Design review of the part built by this model. Coordinates are the model's own, in mm. Face numbers are marked on the shaded views. A direction names the side the tool comes from. Coordinates: 2 decimals unless noted, no trailing zeros. Write each loop counter-clockwise with the first axis right and the second up, starting at its lowest first coordinate (ties: lowest second). Pieces come first, ordered by that corner, then holes.
Q1. For probe 1 along Y at (x, z) = (0, -0.25); probe 2 along Y at (x, z) = (0, 6); probe 3 along Z at (x, y) = (1.5, 6), list the stretches that pass through material, from the lowest coordinate up.
Q2. Take a section at D-D (x = 3.5). Give the boundary of the cut face in (y, z).
Q3. Take a section at C-C (z = 6.25). Give the boundary of the cut face in (x, y).
Q4. Take a section at A-A (x = 0). Give the boundary of the cut face in (y, z), and give its area (3 significant figures).
Q5. Mouldability with a two-part tool opening along Y and no side actions: class the marked faces 3, 4 and 5 as pulls with the +Y half, pulls with the -Y half, needs draft (parallel to the pull), parting line crosses it, or undercut.
Q6. Machinability: for the marked faces 1 and 2, which of the approach directions +Z, -Z, +X, -X, +Y, -Y give a long, thin tool a straight path to every point of the face, cutting with its end or side? Answer none if there is none.
Q7. Insertion check: pin 1 (1.5 mm diameter, centred on x = 2.5, z = 4, fed in from -Y); pin 2 (5 mm diameter, centred on y = 1.5, z = 13, fed in from -X); pin 3 (4 mm diameter, centred on y = -6.5, z = 7, fed in from -X); pin 4 (5 mm diameter, centred on x = 0, y = 0, fed in from -Z). Each pin has a flat end and moves straight along its axis. Give the tip position at first contact, or say it passes through.
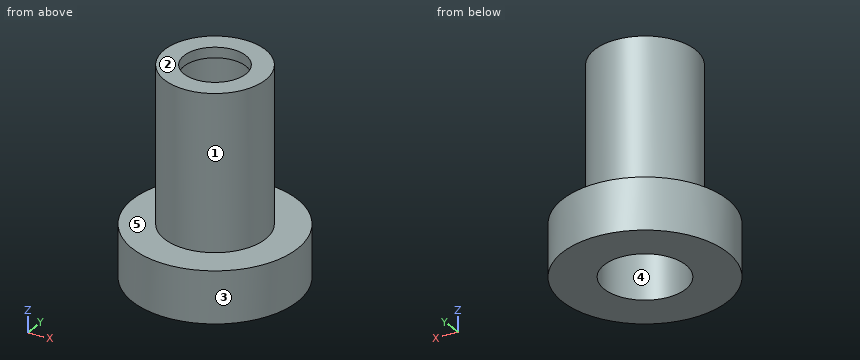
```python
from build123d import *

# Parameters (mm, degrees)
F0_R          = 4.9
F1_DEPTH      = 14
F2_R          = 8
F3_DEPTH      = 5
F4_R          = 3.95
F5_DEPTH      = 25
F5_DEPTH_BACK = 25
F7_R          = 4.9
F7_R_2        = 3
F8_DEPTH      = 1


with BuildPart() as f1:
    # F0 (on Top) → F1 (new body)
    with BuildSketch(Plane.XY):
        Circle(F0_R)
    extrude(amount=F1_DEPTH)

    # F2 (on Top) → F3 (join)
    with BuildSketch(Plane.XY):
        Circle(F2_R)
    extrude(amount=-F3_DEPTH)

    # F4 (on Top) → F5 (cut, two sides)
    with BuildSketch(Plane.XY) as f5_sk:
        Circle(F4_R)
    extrude(amount=-F5_DEPTH, mode=Mode.SUBTRACT)
    extrude(f5_sk.sketch, amount=F5_DEPTH_BACK, mode=Mode.SUBTRACT)

    # F7 (on offset) → F8 (join)
    with BuildSketch(Plane.XY.offset(14)):
        Circle(F7_R)
        Circle(F7_R_2, mode=Mode.SUBTRACT)
    extrude(amount=F8_DEPTH)


solid = f1.part
```
Response:
1. probe 1: y = -8 to -3.95, 3.95 to 8
1. probe 2: y = -4.9 to -3.95, 3.95 to 4.9
1. probe 3: z = -5 to 0
2. outline: (-7.19, -5) - (-1.83, -5) - (-1.83, 14) - (1.83, 14) - (1.83, -5) - (7.19, -5) - (7.19, 0) - (3.43, 0) - (3.43, 15) - (-3.43, 15) - (-3.43, 0) - (-7.19, 0) - close
3. outline: circle Ø9.8 at (0, 0); hole circle Ø7.9 at (0, 0)
4. outline: (-8, -5) - (-3.95, -5) - (-3.95, 14) - (-3, 14) - (-3, 15) - (-4.9, 15) - (-4.9, 0) - (-8, 0) - close; (3, 14) - (3.95, 14) - (3.95, -5) - (8, -5) - (8, 0) - (4.9, 0) - (4.9, 15) - (3, 15) - close
4. area: 70.9 mm2
5. face 3: parting line crosses it
5. face 4: undercut
5. face 5: needs draft
6. face 1: +Z
6. face 2: +Z, +X, -X, +Y, -Y
7. pin 1: stops at y = -4.58
7. pin 2: stops at x = -4.9
7. pin 3: stops at x = -1.94
7. pin 4: passes through
